```python
from build123d import *

# Parameters (mm, degrees)
SKETCH1_R           = 1
SKETCH1_R_2         = 3.5
BOSS_EXTRUDE2_DEPTH = 2.5
SKETCH2_R           = 1
SKETCH2_W           = 20
SKETCH2_H           = 3
CUT_EXTRUDE1_DEPTH  = 34.395358959


with BuildPart() as part:
    # Sketch1 → Boss-Extrude2 (new, symmetric)
    with BuildSketch(Plane.XY):
        with BuildLine():
            Line((7.5, 15), (15, 15))
            ThreePointArc((15, 15), (17.5, 17.5), (15, 20))
            Line((15, 20), (8, 20))
            ThreePointArc((8, 20), (0, 28), (-8, 20))
            Line((-8, 20), (-15, 20))
            ThreePointArc((-15, 20), (-17.5, 17.5), (-15, 15))
            Line((-15, 15), (-7.5, 15))
            Line((-7.5, 15), (-7.5, -15))
            Line((-7.5, -15), (-15, -15))
            ThreePointArc((-15, -15), (-17.5, -17.5), (-15, -20))
            Line((-15, -20), (15, -20))
            ThreePointArc((15, -20), (17.5, -17.5), (15, -15))
            Line((15, -15), (7.5, -15))
            Line((7.5, -15), (7.5, 15))
        make_face()
        with Locations((-15, 17.5)):
            Circle(SKETCH1_R, mode=Mode.SUBTRACT)
        with Locations((15, 17.5)):
            Circle(SKETCH1_R, mode=Mode.SUBTRACT)
        with Locations(Location((15, -17.5, 0), (0, 0, 180))):
            Circle(SKETCH1_R, mode=Mode.SUBTRACT)
        with Locations(Location((-15, -17.5, 0), (0, 0, 180))):
            Circle(SKETCH1_R, mode=Mode.SUBTRACT)
        with Locations((0, 20)):
            Circle(SKETCH1_R_2, mode=Mode.SUBTRACT)
    extrude(amount=BOSS_EXTRUDE2_DEPTH, both=True)

    # Sketch2 → Cut-Extrude1 (cut, through all)
    with BuildSketch(Plane.XY.offset(2.5)):
        Circle(SKETCH2_R)
        with Locations((0, 17.5)):
            Rectangle(SKETCH2_W, SKETCH2_H)
        with Locations((0, -17.5)):
            Rectangle(SKETCH2_W, SKETCH2_H)
    extrude(amount=-CUT_EXTRUDE1_DEPTH, mode=Mode.SUBTRACT)


solid = part.part
```
Check sheet for the modelled part. Datum: model origin and axes. Units: mm. A direction names the side the tool comes from. Give positions to 0.01 mm unless a question says otherwise; leave off trailing zeros. Write each loop counter-clockwise with the first axis right and the second up, starting at its lowest first coordinate (ties: lowest second). Pieces come first, ordered by that corner, then holes. Notation, with made-up numbers: (21, 56.25) - (35, 56.25) arc R28 ccw to (35, 86.25) - close; hole circle Ø10 at (79, 13.25). An arc over 180 degrees is marked (long way). Answer as a JSON object with one key per item and string values. Group by question number.
1) Sectioned sample at A-A (y = 0). Record the cut outline in (x, z), then the cut area to 3 significant figures.
2) Depth check by flat-ended pin: P1, Ø2, axis at y = -11, z = -1, coming from the -X side; P2, Ø3, axis at x = -3.5, z = 2, coming from the +Y side; P3, Ø1.6, axis at x = -15, y = -17.5, coming from the -Z side; P4, Ø2.5, axis at x = -10, z = -1, coming from the +Y side. Enter the tip coordinate at first touch or a pass-through.
3) Thickness scan on probe 1 along Y at (x, z) = (0, -0.05); probe 2 along Y at (x, z) = (-15, 1.2); probe 3 along Y at (x, z) = (11, 0.1). Record the ranges inside material, lowest first. Write a range as from..to.
4) Sectioned sample at D-D (y = 17.5). Record the cut outline in (x, z).
5) Access from +Z, -Z, +X, -X, +Y, -Y to the whole of each face (thin tool, end or side, straight path). Record for faces 1 (the face through (-7.5, 0, 0)), 2 (the face through (0, 4, 2.5)), 3 (the face through (11, -15, 0)), 4 (the face through (10, -18, 0)).
6) Release check for a two-part mould opening along Y. For faces 5 (the face through (0, 28, 0)), 6 (the face through (0, 4, -2.5)), 7 (the face through (0.1, 23.5, 0)), 8 (the face through (-10, -18, 0)) record: pulls with the +Y half, pulls with the -Y half, needs draft (parallel to the pull), parting line crosses it, or undercut.
7) Sectioned sample at C-C (x = 0). Record the cut outline in (y, z).
8) Sectioned sample at B-B (z = -0.25). Give the number of separate pieces and of enclosed holes in the cut face, then the cut area to 3 significant figures.
Geometry results:
{
 "1": {"outline": "(-7.5, -2.5) - (-1, -2.5) - (-1, 2.5) - (-7.5, 2.5) - close; (1, -2.5) - (7.5, -2.5) - (7.5, 2.5) - (1, 2.5) - close", "area": "65.0 mm^2"},
 "2": {"P1": "stops at x = -7.5", "P2": "stops at y = 27.75", "P3": "passes through", "P4": "stops at y = 20"},
 "3": {"probe 1": "y = -20..-19, -16..-1, 1..16, 23.5..28", "probe 2": "y = -20..-18.5, -16.5..-15, 15..16.5, 18.5..20", "probe 3": "y = -20..-15, 15..20"},
 "4": {"outline": "(-17.5, -2.5) - (-16, -2.5) - (-16, 2.5) - (-17.5, 2.5) - close; (-14, -2.5) - (-10, -2.5) - (-10, 2.5) - (-14, 2.5) - close; (10, -2.5) - (14, -2.5) - (14, 2.5) - (10, 2.5) - close; (16, -2.5) - (17.5, -2.5) - (17.5, 2.5) - (16, 2.5) - close"},
 "5": {"face 1": "+Z, -Z, -X", "face 2": "+Z, +X, -X, +Y, -Y", "face 3": "+Z, -Z, +X", "face 4": "+Z, -Z"},
 "6": {"face 5": "pulls with the +Y half", "face 6": "needs draft", "face 7": "undercut", "face 8": "undercut"},
 "7": {"outline": "(-20, -2.5) - (-19, -2.5) - (-19, 2.5) - (-20, 2.5) - close; (-16, -2.5) - (-1, -2.5) - (-1, 2.5) - (-16, 2.5) - close; (1, -2.5) - (16, -2.5) - (16, 2.5) - (1, 2.5) - close; (23.5, -2.5) - (28, -2.5) - (28, 2.5) - (23.5, 2.5) - close"},
 "8": {"separate pieces": "1", "enclosed holes": "7", "area": "728 mm^2"}
}
